```python
from build123d import *

# Parameters (mm, degrees)
SKETCH_1_R      = 0.499999
EXTRUDE_1_DEPTH = 0.41148


with BuildPart() as part:
    # 草图1 → 凸台-拉伸1 (new body)
    with BuildSketch(Plane.XY):
        Polygon((-23.99008664, 0.03617468), (-23.50000126, -0.01209548), (-23.50000126, 0), (-2.50000008, -0.01209548), (-2.0099147, 0.03617468), (-1.53866342, 0.17912588), (-1.1043539, 0.41126918), (-0.72367902, 0.72367902), (-0.41126918, 1.1043539), (-0.17912588, 1.53866342), (-0.03617468, 2.0099147), (0.01209548, 2.50000008), (-1.27e-05, 2.50000008), (-1.27e-05, 17.50001326), (0.01209548, 17.50000056), (-0.03617468, 17.99008594), (-0.17912588, 18.46133722), (-0.41126918, 18.89564674), (-0.72367902, 19.27632162), (-1.1043539, 19.58873146), (-1.53866342, 19.82087476), (-2.0099147, 19.96382596), (-2.50000008, 20.01209612), (-2.50000008, 20.000013333), (-23.492043121, 20.012146936), (-23.98367568, 19.9637269), (-24.45643572, 19.82031596), (-24.89213462, 19.58743098), (-25.27402616, 19.27401784), (-25.5874393, 18.8921263), (-25.82032428, 18.4564274), (-25.96373522, 17.98366736), (-26.01215524, 17.49201734), (-26.0000115, 17.49201734), (-26.0000115, 2.50001278), (-26.01209682, 2.50000008), (-25.96382666, 2.0099147), (-25.82087546, 1.53866342), (-25.58873216, 1.1043539), (-25.27632232, 0.72367902), (-24.89564744, 0.41126918), (-24.46133792, 0.17912588), align=None)
        with Locations(Location((-23.1599867, 17.74997974, 0), (0, 0, 180))):
            Circle(SKETCH_1_R, mode=Mode.SUBTRACT)
        with Locations(Location((-20.6199867, 17.74997974, 0), (0, 0, 180))):
            Circle(SKETCH_1_R, mode=Mode.SUBTRACT)
        with Locations(Location((-20.6199867, 2.24998534, 0), (0, 0, 180))):
            Circle(SKETCH_1_R, mode=Mode.SUBTRACT)
        with Locations(Location((-15.5399867, 17.74997974, 0), (0, 0, 180))):
            Circle(SKETCH_1_R, mode=Mode.SUBTRACT)
        with Locations(Location((-12.9999867, 17.74997974, 0), (0, 0, 180))):
            Circle(SKETCH_1_R, mode=Mode.SUBTRACT)
        with Locations(Location((-18.0799867, 17.74997974, 0), (0, 0, 180))):
            Circle(SKETCH_1_R, mode=Mode.SUBTRACT)
        with Locations(Location((-18.0799867, 2.24998534, 0), (0, 0, 180))):
            Circle(SKETCH_1_R, mode=Mode.SUBTRACT)
        with Locations(Location((-15.5399867, 2.24998534, 0), (0, 0, 180))):
            Circle(SKETCH_1_R, mode=Mode.SUBTRACT)
        with Locations(Location((-23.1599867, 2.24998534, 0), (0, 0, 180))):
            Circle(SKETCH_1_R, mode=Mode.SUBTRACT)
        with Locations(Location((-10.4599867, 2.24998534, 0), (0, 0, 180))):
            Circle(SKETCH_1_R, mode=Mode.SUBTRACT)
        with Locations(Location((-12.9999867, 2.24998534, 0), (0, 0, 180))):
            Circle(SKETCH_1_R, mode=Mode.SUBTRACT)
        with Locations(Location((-7.9199867, 17.74997974, 0), (0, 0, 180))):
            Circle(SKETCH_1_R, mode=Mode.SUBTRACT)
        with Locations(Location((-5.3799867, 17.74997974, 0), (0, 0, 180))):
            Circle(SKETCH_1_R, mode=Mode.SUBTRACT)
        with Locations(Location((-10.4599867, 17.74997974, 0), (0, 0, 180))):
            Circle(SKETCH_1_R, mode=Mode.SUBTRACT)
        with Locations(Location((-2.8399867, 17.74997974, 0), (0, 0, 180))):
            Circle(SKETCH_1_R, mode=Mode.SUBTRACT)
        with Locations(Location((-1.49999954, 13.03999932, 0), (0, 0, 180))):
            Circle(SKETCH_1_R, mode=Mode.SUBTRACT)
        with Locations(Location((-5.3799867, 2.24998534, 0), (0, 0, 180))):
            Circle(SKETCH_1_R, mode=Mode.SUBTRACT)
        with Locations(Location((-2.8399867, 2.24998534, 0), (0, 0, 180))):
            Circle(SKETCH_1_R, mode=Mode.SUBTRACT)
        with Locations(Location((-7.9199867, 2.24998534, 0), (0, 0, 180))):
            Circle(SKETCH_1_R, mode=Mode.SUBTRACT)
        with Locations(Location((-1.49999954, 10.49999932, 0), (0, 0, 180))):
            Circle(SKETCH_1_R, mode=Mode.SUBTRACT)
        with Locations(Location((-1.49999954, 7.95999932, 0), (0, 0, 180))):
            Circle(SKETCH_1_R, mode=Mode.SUBTRACT)
    extrude(amount=-EXTRUDE_1_DEPTH)


solid = part.part
```
Source: CAD feature listing. Evaluate the final solid. Frame: model axes, mm. Give positions to 0.01 mm unless a question says otherwise; leave off trailing zeros. Loops run counter-clockwise (first coordinate to the right, second up) from the corner with the lowest first, then second, coordinate; pieces in that order, holes last. Notation, with made-up numbers: (61.5, -17.5) -> (78.5, -17.5) arc R22 cw to (78.5, -10.5) -> close; hole circle Ø3 at (11, 34.5). An arc over 180 degrees is marked (long way). Use a Markdown table: item, result. Add a question column.
(1) Pull-direction query (X, two-part tool) for faces 1 (the face through (-13, 10, 0)), 2 (the face through (-18.3, 17.3, -0.2)); classes: +X half, -X half, draft (parallel to the pull), parting line (faces both ways), or undercut.
(2) Section query A-A (y = 13.04). Output: boundary loops of the cut face in (x, z).
(3) Section query B-B (z = -0.3). Count the separate pieces of the cut face and the enclosed holes in it, then the cut area to 3 significant figures.
(4) Ray query, line 1 (X direction, y = 13, z = -0.1); line 2 (X direction, y = 12, z = -0.05); line 3 (Y direction, x = -4.5, z = -0.1). Return the intervals inside material, ascending.
Checked values:
| question | item | result |
|---|---|---|
| 1 | face 1 | draft |
| 1 | face 2 | undercut |
| 2 | outline | (-26, -0.41) -> (-2, -0.41) -> (-2, 0) -> (-26, 0) -> close; (-1, -0.41) -> (0, -0.41) -> (0, 0) -> (-1, 0) -> close |
| 3 | separate pieces | 1 |
| 3 | enclosed holes | 21 |
| 3 | area | 498 mm^2 |
| 4 | line 1 | -26 to -2, -1 to 0 |
| 4 | line 2 | -26 to 0 |
| 4 | line 3 | -0.01 to 20 |
